Verification items for this drawing (mm, ordinates from the low corner). A direction names the side the tool comes from. Round coordinates to 2 decimals unless told otherwise and drop trailing zeros. Order: outer loops, then holes, each group sorted by start corner. A loop starts at its lowest first (then second) coordinate and runs counter-clockwise, first axis right, second up. Notation, with made-up numbers: (-23.5, 19) -> (28.5, 19) arc R23 ccw to (28.5, 53) -> close; hole circle Ø6 at (80.5, 51.5). An arc over 180 degrees is marked (long way). Put each result on its own line as item: value.
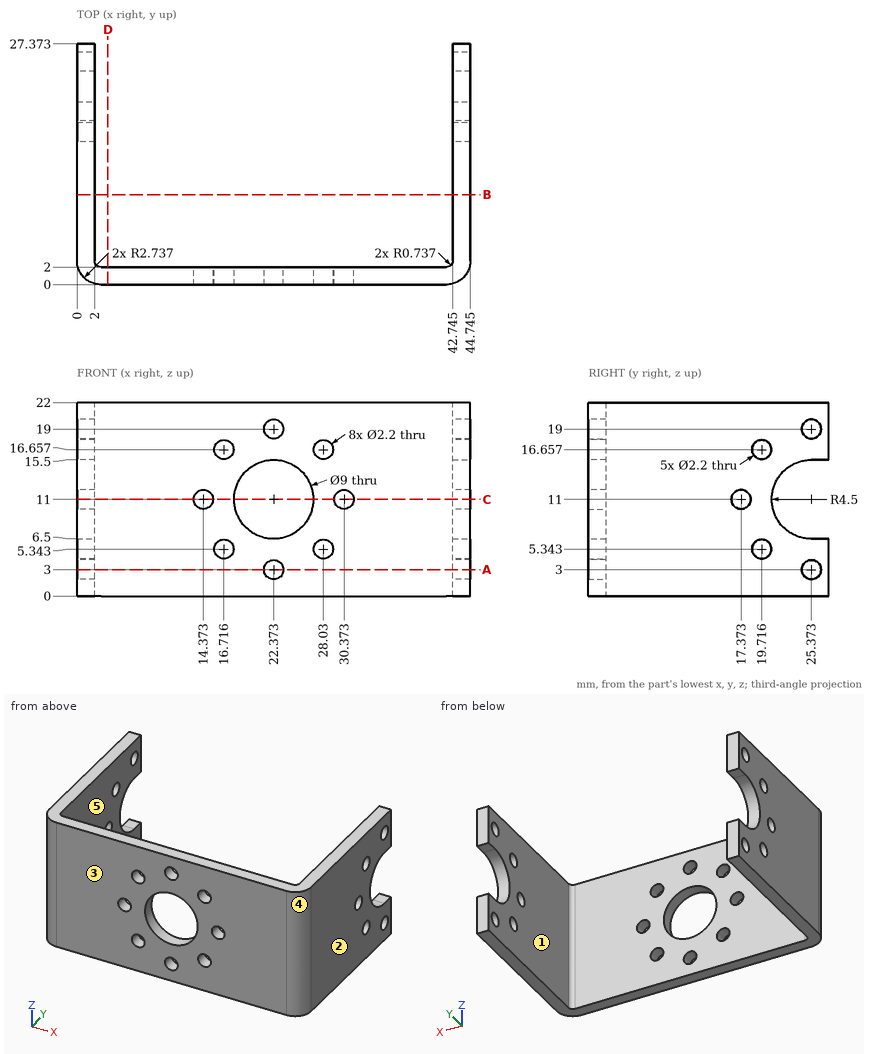
Item 1: Section check B-B on y = 10.25. Record the boundary of the cut face in (x, z) (1 decimal).
Check sheet entries:
outline: (0, 0) -> (2, 0) -> (2, 22) -> (0, 22) -> close; (42.7, 0) -> (44.7, 0) -> (44.7, 22) -> (42.7, 22) -> close
Item 2: Section check C-C on z = 11. State how many separate pieces and enclosed holes the cut face has.
Check sheet entries:
separate pieces: 6
enclosed holes: 0
Item 3: Tool access check on the marked faces 4 and 5. Record the directions out of +Z, -Z, +X, -X, +Y, -Y that give a thin tool (end or side, any length) a straight path to the whole face; none if there is none.
Check sheet entries:
face 4: +Z, -Z, +X, -Y
face 5: +Z, -Z, +Y
Item 4: Release check for a two-part mould opening along X. For the marked faces 1, 2 and 3 record: +X half, -X half, draft (parallel to the pull), parting line (faces both ways), or undercut.
Check sheet entries:
face 1: undercut
face 2: +X half
face 3: draft
Item 5: Material ranges on L1, parallel to X at y = 5.5, z = 20.5 (1 decimal); L2, parallel to Z at x = 23, y = 1.75 (1 decimal); L3, parallel to Y at x = 7.5, z = 7, recorded low to high. Write a range as [from, to].
Check sheet entries:
L1: x = [0, 2], [42.7, 44.7]
L2: z = [0, 2.1], [3.9, 6.5], [15.5, 18.1], [19.9, 22]
L3: y = [0, 2]
Item 6: Gauge pin test, flat end, axial feed: pin 1 Ø1.8 at (y, z) = (25.37, 19) entering from -X. Record the tip position at first contact, or that the pin passes through.
Check sheet entries:
pin 1: passes through
Item 7: Section check D-D on x = 3.5. Record the boundary of the cut face in (y, z).
Check sheet entries:
outline: (0, 0) -> (2, 0) -> (2, 22) -> (0, 22) -> close
Item 8: Section check A-A on z = 3. Record the boundary of the cut face in (x, y) (1 decimal).
Check sheet entries:
outline: (0, 2.7) arc R2.7 ccw to (2.7, 0) -> (21.3, 0) -> (21.3, 2) -> (2.7, 2) arc R0.7 cw to (2, 2.7) -> (2, 24.3) -> (0, 24.3) -> close; (0, 26.5) -> (2, 26.5) -> (2, 27.4) -> (0, 27.4) -> close; (23.5, 0) -> (42, 0) arc R2.7 ccw to (44.7, 2.7) -> (44.7, 24.3) -> (42.7, 24.3) -> (42.7, 2.7) arc R0.7 cw to (42, 2) -> (23.5, 2) -> close; (42.7, 26.5) -> (44.7, 26.5) -> (44.7, 27.4) -> (42.7, 27.4) -> close
